```python
from build123d import *

# Parameters (mm, degrees)
F0_W     = 100
F0_H     = 92.5255602876
F1_DEPTH = 10
F2_DEPTH = 3
F3_DEPTH = 6
F4_R     = 3


with BuildPart() as f1:
    # F0 (on Top) → F1 (new body)
    with BuildSketch(Plane.XY):
        Rectangle(F0_W, F0_H)
        with BuildLine():
            ThreePointArc((-13.8530512527, -41.8971102989), (0, 44.1279376406), (13.8530512527, -41.8971102989))
            Line((13.8530512527, -41.8971102989), (2.9358495271, -13.4106839777))
            ThreePointArc((2.9358495271, -13.4106839777), (0, 13.7282794696), (-2.9358495271, -13.4106839777))
            Line((-2.9358495271, -13.4106839777), (-13.8530512527, -41.8971102989))
        make_face(mode=Mode.SUBTRACT)
        with BuildLine():
            Line((2.9358495271, -13.4106839777), (13.8530512527, -41.8971102989))
            ThreePointArc((13.8530512527, -41.8971102989), (0, 44.1279376406), (-13.8530512527, -41.8971102989))
            Line((-13.8530512527, -41.8971102989), (-2.9358495271, -13.4106839777))
            ThreePointArc((-2.9358495271, -13.4106839777), (0, 13.7282794696), (2.9358495271, -13.4106839777))
        make_face()
        with BuildLine():
            ThreePointArc((-16.157050142, -36.7314730169), (0, 40.1279376406), (16.157050142, -36.7314730169))
            Line((16.157050142, -36.7314730169), (7.8820297495, -15.1393320411))
            ThreePointArc((7.8820297495, -15.1393320411), (0, 17.0682678566), (-7.8820297495, -15.1393320411))
            Line((-7.8820297495, -15.1393320411), (-16.157050142, -36.7314730169))
        make_face(mode=Mode.SUBTRACT)
        with BuildLine():
            Line((7.8820297495, -15.1393320411), (16.157050142, -36.7314730169))
            ThreePointArc((16.157050142, -36.7314730169), (0, 40.1279376406), (-16.157050142, -36.7314730169))
            Line((-16.157050142, -36.7314730169), (-7.8820297495, -15.1393320411))
            ThreePointArc((-7.8820297495, -15.1393320411), (0, 17.0682678566), (7.8820297495, -15.1393320411))
        make_face()
    extrude(amount=-F1_DEPTH)

    # F0 (on Top) → F2 (join)
    with BuildSketch(Plane.XY):
        with BuildLine():
            Line((2.9358495271, -13.4106839777), (13.8530512527, -41.8971102989))
            ThreePointArc((13.8530512527, -41.8971102989), (0, 44.1279376406), (-13.8530512527, -41.8971102989))
            Line((-13.8530512527, -41.8971102989), (-2.9358495271, -13.4106839777))
            ThreePointArc((-2.9358495271, -13.4106839777), (0, 13.7282794696), (2.9358495271, -13.4106839777))
        make_face()
        with BuildLine():
            ThreePointArc((-16.157050142, -36.7314730169), (0, 40.1279376406), (16.157050142, -36.7314730169))
            Line((16.157050142, -36.7314730169), (7.8820297495, -15.1393320411))
            ThreePointArc((7.8820297495, -15.1393320411), (0, 17.0682678566), (-7.8820297495, -15.1393320411))
            Line((-7.8820297495, -15.1393320411), (-16.157050142, -36.7314730169))
        make_face(mode=Mode.SUBTRACT)
        with BuildLine():
            Line((7.8820297495, -15.1393320411), (16.157050142, -36.7314730169))
            ThreePointArc((16.157050142, -36.7314730169), (0, 40.1279376406), (-16.157050142, -36.7314730169))
            Line((-16.157050142, -36.7314730169), (-7.8820297495, -15.1393320411))
            ThreePointArc((-7.8820297495, -15.1393320411), (0, 17.0682678566), (7.8820297495, -15.1393320411))
        make_face()
    extrude(amount=F2_DEPTH)

    # F0 (on Top) → F3 (join)
    with BuildSketch(Plane.XY):
        with BuildLine():
            Line((7.8820297495, -15.1393320411), (16.157050142, -36.7314730169))
            ThreePointArc((16.157050142, -36.7314730169), (0, 40.1279376406), (-16.157050142, -36.7314730169))
            Line((-16.157050142, -36.7314730169), (-7.8820297495, -15.1393320411))
            ThreePointArc((-7.8820297495, -15.1393320411), (0, 17.0682678566), (7.8820297495, -15.1393320411))
        make_face()
    extrude(amount=F3_DEPTH)

    # F4
    f4_edges = [f1.edges().sort_by_distance(p)[0] for p in [
        (-2.93585, -13.410684, 1.5),
        (2.93585, -13.410684, 1.5),
        (13.853051, -41.89711, 1.5),
        (-13.853051, -41.89711, 1.5),
    ]]
    fillet(f4_edges, radius=F4_R)


solid = f1.part
```
The model under review builds one solid part; all positions refer to its coordinate system, in mm. A direction names the side the tool comes from. Coordinates: 2 decimals unless noted, no trailing zeros. Order: outer loops, then holes, each group sorted by start corner. A loop starts at its lowest first (then second) coordinate and runs counter-clockwise, first axis right, second up. Notation, with made-up numbers: M -31,-39.5 L -10,-39.5 A20 ccw -10,-19.5 Z; hole C -11,-13.5 d6. An arc over 180 degrees is marked long. One line per question, with ' | ' between items.
(1) Machinability: for faces 1 (the face through (-1, 1, 0)), 2 (the face through (-1, 1, -10)), 3 (the face through (14.373, -40.797, 1.521)), which of the approach directions +Z, -Z, +X, -X, +Y, -Y give a long, thin tool a straight path to every point of the face, cutting with its end or side? Answer none if there is none.
Geometry results:
face 1: +Z | face 2: -Z, +X, -X, +Y, -Y | face 3: +Z, -Y
(2) Add section A-A, the plane x = 0. Write out the cut boundary in (y, z).
Geometry results:
outline: M -46.26,-10 L 46.26,-10 L 46.26,0 L 44.13,0 L 44.13,3 L 40.13,3 L 40.13,6 L 17.07,6 L 17.07,3 L 13.73,3 L 13.73,0 L -46.26,0 Z
(3) For probe 1 along X at (y, z) = (0, 1.2); probe 2 along X at (y, z) = (0, 4.7); probe 3 along Y at (x, z) = (0, 4.05), list the stretches that pass through material, from the lowest coordinate up. Write a range as from..to.
Geometry results:
probe 1: x = -44.13..-13.73, 13.73..44.13 | probe 2: x = -40.13..-17.07, 17.07..40.13 | probe 3: y = 17.07..40.13
(4) Add section B-B, the plane y = 0. Write out the cut boundary in (x, z), then the cut area to 3 significant figures.
Geometry results:
outline: M -50,-10 L 50,-10 L 50,0 L 44.13,0 L 44.13,3 L 40.13,3 L 40.13,6 L 17.07,6 L 17.07,3 L 13.73,3 L 13.73,0 L -13.73,0 L -13.73,3 L -17.07,3 L -17.07,6 L -40.13,6 L -40.13,3 L -44.13,3 L -44.13,0 L -50,0 Z | area: 1,320 mm²
(5) Add section D-D, the plane y = -28.5. Write out the cut boundary in (x, z), then the cut area to 3 significant figures.
Geometry results:
outline: M -50,-10 L 50,-10 L 50,0 L 33.69,0 L 33.69,3 L 28.25,3 L 28.25,6 L 13,6 L 13,3 L 8.72,3 L 8.72,0 L -8.72,0 L -8.72,3 L -13,3 L -13,6 L -28.25,6 L -28.25,3 L -33.69,3 L -33.69,0 L -50,0 Z | area: 1,240 mm²
(6) Add section C-C, the plane x = -19.5. Write out the cut boundary in (y, z), then the cut area to 3 significant figures.
Geometry results:
outline: M -46.26,-10 L 46.26,-10 L 46.26,0 L 39.59,0 L 39.59,3 L 35.07,3 L 35.07,6 L -35.07,6 L -35.07,3 L -39.59,3 L -39.59,0 L -46.26,0 Z | area: 1,370 mm²
(7) Insertion check: pin 1 (1 mm diameter, centred on x = 28.5, z = 2.5, fed in from +Y). The pin has a flat end and moves straight along its axis. Give the tip position at first contact, or say it passes through.
Geometry results:
pin 1: stops at y = 34.11
(8) The part is to be moulded in two halves that separate along X. For faces 4 (the face through (-14.43, -40.82, 1.52)), 5 (the face through (-1, -46.263, -5)), 6 (the face through (1.5, 40.1, 4.5)), say which applies: +X half, -X half, draft (parallel to the pull), parting line (faces both ways), or undercut.
Geometry results:
face 4: undercut | face 5: draft | face 6: parting line
